from build123d import *

# Parameters (mm, degrees)
Y_KSEKLIK_EKSTR_ZYON1_DEPTH = 500
RADYUS1_R                   = 2
IZIM2_R                     = 4.25
KES_EKSTR_ZYON1_DEPTH       = 10
PAH1_SIZE                   = 3


with BuildPart() as part:
    # Çizim1 → Yükseklik-Ekstrüzyon1 (new body)
    with BuildSketch(Plane.XY):
        Polygon((0, 0), (65, 0), (65, 4), (10, 4), (10, 8), (5, 8), (5, 4), (0, 4), align=None)
    extrude(amount=-Y_KSEKLIK_EKSTR_ZYON1_DEPTH)

    # Radyus1
    radyus1_edges = [part.edges().sort_by_distance(p)[0] for p in [
        (5, 8, -250),
        (10, 8, -250),
    ]]
    fillet(radyus1_edges, radius=RADYUS1_R)

    # Çizim2 → Kes-Ekstrüzyon1 (cut)
    with BuildSketch(Plane.XZ):
        with Locations(Location((30, -40, 0), (0, 0, 270))):
            Circle(IZIM2_R)
        with Locations(Location((30, -180, 0), (0, 0, 270))):
            Circle(IZIM2_R)
        with Locations(Location((30, -320, 0), (0, 0, 270))):
            Circle(IZIM2_R)
        with Locations(Location((30, -460, 0), (0, 0, 270))):
            Circle(IZIM2_R)
    extrude(amount=-KES_EKSTR_ZYON1_DEPTH, mode=Mode.SUBTRACT)

    # Pah1
    pah1_edges = [part.edges().sort_by_distance(p)[0] for p in [
        (30, 4, -35.75),
        (30, 4, -175.75),
        (30, 4, -315.75),
        (30, 4, -455.75),
    ]]
    chamfer(pah1_edges, length=PAH1_SIZE)


solid = part.part
Geometry: final body of the model. Coordinates: model frame, mm. A direction names the side the tool comes from. Give positions to 0.01 mm unless a question says otherwise; leave off trailing zeros. Loops run counter-clockwise (first coordinate to the right, second up) from the corner with the lowest first, then second, coordinate; pieces in that order, holes last. Notation, with made-up numbers: (-22.75, 72.25) - (9.25, 72.25) arc R19 ccw to (9.25, 97.25) - close; hole circle Ø3 at (-0.75, 82.25). An arc over 180 degrees is marked (long way). Answer as CSV lines item,"result". Start each with the question number.
1. Section A-A, the plane x = 30. Return loops of the section in (y, z), plus the area to 3 significant figures.
2. Section C-C, the plane z = -214. Return loops of the section in (x, y), plus the area to 3 significant figures.
3. Draft query along Z for faces 1 (the face through (28.316, 1.146, -464.06)), 2 (the face through (32, 1, -500)), 3 (the face through (32, 1, 0)), 4 (the face through (32, 0, -246)). Return one class per face: released by +Z, released by -Z, zero draft, split by the parting line, or undercut.
4. Reachability of faces 5 (the face through (38, 4, -246)), 6 (the face through (30.187, 0.493, -35.754)) from +Z, -Z, +X, -X, +Y, -Y: full face, straight path, thin tool, end or side. Return the list, or none.
5. Section B-B, the plane z = -460. Return loops of the section in (x, y), plus the area to 3 significant figures.
6. Pin query (flat end, axial travel): P1, Ø4, axis at x = 3.5, z = -311, coming from the +Y side; P2, Ø10, axis at x = 30, z = -460, coming from the +Y side; P3, Ø2, axis at y = 5.5, z = -254.5, coming from the -X side. Return the tip coordinate at first contact, or that it passes through.
7. Ray query, L1, parallel to X at y = 0.55, z = -180; L2, parallel to Y at x = 59, z = -268.5; L3, parallel to X at y = 5.25, z = -99.5. Return the intervals inside material, ascending.
Answers:
1,outline,"(0, -500) - (4, -500) - (4, -467.25) - (1, -464.25) - (0, -464.25) - close; (0, -455.75) - (1, -455.75) - (4, -452.75) - (4, -327.25) - (1, -324.25) - (0, -324.25) - close; (0, -315.75) - (1, -315.75) - (4, -312.75) - (4, -187.25) - (1, -184.25) - (0, -184.25) - close; (0, -175.75) - (1, -175.75) - (4, -172.75) - (4, -47.25) - (1, -44.25) - (0, -44.25) - close; (0, -35.75) - (1, -35.75) - (4, -32.75) - (4, 0) - (0, 0) - close"
1,area,"1,830 mm2"
2,outline,"(0, 0) - (65, 0) - (65, 4) - (10, 4) - (10, 6) arc R2 ccw to (8, 8) - (7, 8) arc R2 ccw to (5, 6) - (5, 4) - (0, 4) - close"
2,area,"278 mm2"
3,face 1,"undercut"
3,face 2,"released by -Z"
3,face 3,"released by +Z"
3,face 4,"zero draft"
4,face 5,"+Z, -Z, +X, +Y"
4,face 6,"+Y, -Y"
5,outline,"(0, 0) - (25.75, 0) - (25.75, 1) - (22.75, 4) - (10, 4) - (10, 6) arc R2 ccw to (8, 8) - (7, 8) arc R2 ccw to (5, 6) - (5, 4) - (0, 4) - close; (34.25, 0) - (65, 0) - (65, 4) - (37.25, 4) - (34.25, 1) - close"
5,area,"235 mm2"
6,P1,"stops at y = 7.32"
6,P2,"stops at y = 1.75"
6,P3,"stops at x = 5"
7,L1,"x = 0 to 25.75, 34.25 to 65"
7,L2,"y = 0 to 4"
7,L3,"x = 5 to 10"
